from build123d import *
from build123d.topology import SkipClean

# Parameters (mm, degrees)
SKETCH_1_W                 = 85
SKETCH_1_H                 = 5
EXTRUDE_1_DEPTH            = 8
EXTRUDE_1_2_DEPTH          = 8
SKETCH_1_3_W               = 85
SKETCH_1_3_H               = 20
EXTRUDE_2_DEPTH            = 11
EXTRUDE_3_DEPTH            = 21
SKETCH_6_R                 = 6.5
SKETCH_6_R_2               = 4
CUT_EXTRUDE_1_DEPTH        = 3
SKETCH_6_2_R               = 4
CUT_EXTRUDE_2_DEPTH        = 21
EXTRUDE_6_DEPTH            = 20
EXTRUDE_7_DEPTH            = 15
SKETCH_10_4_W              = 15
SKETCH_10_4_H              = 4
CUT_EXTRUDE_4_DEPTH        = 15
CUT_EXTRUDE_2_2_DEPTH      = 66.048059256
CUT_EXTRUDE_2_2_DEPTH_BACK = 1
CUT_EXTRUDE_2_2_START      = 25
SKETCH_12_W                = 2
SKETCH_12_H                = 40
CUT_EXTRUDE_5_REACH        = 59.985
SKETCH_6_4_R               = 4
CUT_EXTRUDE_6_DEPTH        = 81.357015954


with BuildPart() as part:
    # Sketch 1 → Extrude 1 (new body)
    with BuildSketch(Plane(origin=(0, 0, 0), x_dir=(1, 0, 0), z_dir=(0, 1, 0))):
        with Locations((0, 12.5)):
            Rectangle(SKETCH_1_W, SKETCH_1_H)
    extrude(amount=EXTRUDE_1_DEPTH)



with BuildPart() as body_2:
    # Sketch 1 → Extrude 1 2 (new body)
    with BuildSketch(Plane(origin=(0, 0, 0), x_dir=(1, 0, 0), z_dir=(0, 1, 0))):
        with Locations((0, -12.5)):
            Rectangle(SKETCH_1_W, SKETCH_1_H)
    extrude(amount=EXTRUDE_1_2_DEPTH)


with BuildPart() as part_1:
    add(part.part)

    add(body_2.part)  # Extrude 2 merges body 2
    # Sketch 1_3 → Extrude 2 (add)
    with BuildSketch(Plane(origin=(0, 0, 0), x_dir=(1, 0, 0), z_dir=(0, 1, 0))):
        Rectangle(SKETCH_1_3_W, SKETCH_1_3_H)
    extrude(amount=EXTRUDE_2_DEPTH)

    # Sketch 3 → Extrude 3 (add, symmetric)
    with BuildSketch(Plane(origin=(0, 0, 0), x_dir=(0, 0, -1), z_dir=(1, 0, 0))):
        with BuildLine():
            Line((-10, 35), (-10, 11))
            Line((-10, 11), (10, 11))
            Line((10, 11), (10, 35))
            ThreePointArc((10, 35), (0, 45), (-10, 35))
        make_face()
    extrude(amount=EXTRUDE_3_DEPTH, both=True)

    # Sketch 6 → Cut-Extrude 1 (cut)
    with BuildSketch(Plane.ZY.offset(21)):
        with Locations((0, 35)):
            Circle(SKETCH_6_R)
        with Locations((0, 35)):
            Circle(SKETCH_6_R_2, mode=Mode.SUBTRACT)
    cut_extrude_1 = extrude(amount=-CUT_EXTRUDE_1_DEPTH, mode=Mode.SUBTRACT)

    # Sketch 6_2 → Cut-Extrude 2 (cut)
    with BuildSketch(Plane.ZY.offset(21)):
        with Locations((0, 35)):
            Circle(SKETCH_6_2_R)
    cut_extrude_2 = extrude(amount=-CUT_EXTRUDE_2_DEPTH, mode=Mode.SUBTRACT)

    # Mirror 1: Cut-Extrude 1, Cut-Extrude 2 across plane
    add(cut_extrude_1.mirror(Plane(origin=(0, 0, 0), x_dir=(0, 0, 1), z_dir=(1, 0, 0))), mode=Mode.SUBTRACT)
    add(cut_extrude_2.mirror(Plane(origin=(0, 0, 0), x_dir=(0, 0, 1), z_dir=(1, 0, 0))), mode=Mode.SUBTRACT)

    # Sketch 10 → Extrude 6 (add, symmetric)
    with SkipClean():  # the faces are left unmerged after this step: merging them gives an invalid solid
        with BuildSketch(Plane.XY):
            with BuildLine():
                ThreePointArc((15, 25), (10.606601718, 35.606601718), (0, 40))
                Line((0, 40), (0, 33))
                ThreePointArc((0, 33), (5.656854249, 30.656854249), (8, 25))
                ThreePointArc((8, 25), (5.656854249, 19.343145751), (0, 17))
                Line((0, 17), (0, 10))
                ThreePointArc((0, 10), (10.606601718, 14.393398282), (15, 25))
            make_face()
            with BuildLine():
                Line((0, 33), (0, 40))
                ThreePointArc((0, 40), (-10.606601718, 35.606601718), (-15, 25))
                ThreePointArc((-15, 25), (-10.606601718, 14.393398282), (0, 10))
                Line((0, 10), (0, 17))
                ThreePointArc((0, 17), (-8, 25), (0, 33))
            make_face()
        extrude(amount=EXTRUDE_6_DEPTH, both=True)
    add(part_1.part.scale(1), mode=Mode.REPLACE)  # the faces are merged on a copy

    # Sketch 10_3 → Extrude 7 (add, symmetric)
    with BuildSketch(Plane.XY):
        with BuildLine():
            Line((15, 8), (15, 25))
            ThreePointArc((15, 25), (10.606601718, 14.393398282), (0, 10))
            Line((0, 10), (0, 8))
            Line((0, 8), (15, 8))
        make_face()
        with BuildLine():
            ThreePointArc((0, 10), (-10.606601718, 14.393398282), (-15, 25))
            Line((-15, 25), (-15, 8))
            Line((-15, 8), (0, 8))
            Line((0, 8), (0, 10))
        make_face()
    extrude(amount=EXTRUDE_7_DEPTH, both=True)

    # Sketch 10_4 → Cut-Extrude 4 (cut, symmetric)
    with BuildSketch(Plane.XY):
        with BuildLine():
            ThreePointArc((8, 25), (5.656854249, 30.656854249), (0, 33))
            Line((0, 33), (0, 17))
            ThreePointArc((0, 17), (5.656854249, 19.343145751), (8, 25))
        make_face()
        with BuildLine():
            Line((0, 17), (0, 33))
            ThreePointArc((0, 33), (-8, 25), (0, 17))
        make_face()
        with Locations((-7.5, 2)):
            Rectangle(SKETCH_10_4_W, SKETCH_10_4_H)
        with Locations((7.5, 2)):
            Rectangle(SKETCH_10_4_W, SKETCH_10_4_H)
    extrude(amount=CUT_EXTRUDE_4_DEPTH, both=True, mode=Mode.SUBTRACT)

    # Sketch 12 → Cut-Extrude 2 2 (cut, two sides: drawn at the far end of the back side and taken through both)
    with BuildSketch(Plane(origin=(0, 0, 0), x_dir=(1, 0, 0), z_dir=(0, 1, 0)).offset(CUT_EXTRUDE_2_2_START - CUT_EXTRUDE_2_2_DEPTH_BACK)):
        Rectangle(SKETCH_12_W, SKETCH_12_H)
    extrude(amount=CUT_EXTRUDE_2_2_DEPTH + CUT_EXTRUDE_2_2_DEPTH_BACK, mode=Mode.SUBTRACT)

    # Sketch 14 → Cut-Extrude 5 (cut, up to next)
    with BuildSketch(Plane(origin=(0, 11, 0), x_dir=(1, 0, 0), z_dir=(0, 1, 0)), mode=Mode.PRIVATE) as cut_extrude_5_sk1:
        with BuildLine():
            Line((-35, 4), (-30, 4))
            ThreePointArc((-30, 4), (-26, 0), (-30, -4))
            Line((-30, -4), (-35, -4))
            ThreePointArc((-35, -4), (-39, 0), (-35, 4))
        make_face()
    cut_extrude_5_tool1 = extrude(cut_extrude_5_sk1.sketch, amount=-CUT_EXTRUDE_5_REACH, mode=Mode.PRIVATE) & part_1.part
    # Sketch 14 → Cut-Extrude 5 (cut, up to next)
    with BuildSketch(Plane(origin=(0, 11, 0), x_dir=(1, 0, 0), z_dir=(0, 1, 0)), mode=Mode.PRIVATE) as cut_extrude_5_sk2:
        with BuildLine():
            Line((35, 4), (30, 4))
            ThreePointArc((30, 4), (26, 0), (30, -4))
            Line((30, -4), (35, -4))
            ThreePointArc((35, -4), (39, 0), (35, 4))
        make_face()
    cut_extrude_5_tool2 = extrude(cut_extrude_5_sk2.sketch, amount=-CUT_EXTRUDE_5_REACH, mode=Mode.PRIVATE) & part_1.part
    add(cut_extrude_5_tool1.solids().sort_by_distance((-32.5, 11, 0))[0], mode=Mode.SUBTRACT)
    add(cut_extrude_5_tool2.solids().sort_by_distance((32.5, 11, 0))[0], mode=Mode.SUBTRACT)

    # Sketch 6_4 → Cut-Extrude 6 (cut, through all)
    with BuildSketch(Plane.ZY.offset(21)):
        with Locations(Location((0, 35, 0), (0, 0, 328.956646236))):
            Circle(SKETCH_6_4_R)
    extrude(amount=-CUT_EXTRUDE_6_DEPTH, mode=Mode.SUBTRACT)


solid = part_1.part
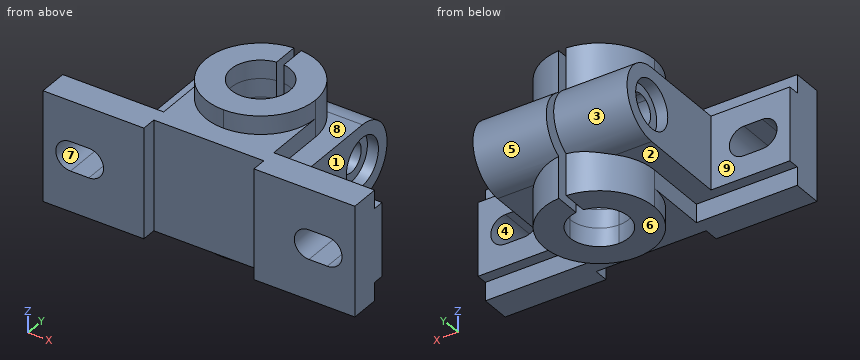
The listing builds one solid part. Answer for the finished solid, in the listing's coordinates (mm). Face numbers are marked on the shaded views. A direction names the side the tool comes from. Round coordinates to 2 decimals unless told otherwise and drop trailing zeros. Order: outer loops, then holes, each group sorted by start corner. A loop starts at its lowest first (then second) coordinate and runs counter-clockwise, first axis right, second up. Notation, with made-up numbers: (1, -29.5) -> (25, -29.5) arc R18 ccw to (25, -2.5) -> close; hole circle Ø6 at (10.25, 89). An arc over 180 degrees is marked (long way). Write each question's results on one line, items separated by ' | '. Start each with the question number.
Q1. Straight lines are drawn through the part: probe 1 along X at (y, z) = (36, -7.5); probe 2 along X at (y, z) = (35, 4.5); probe 3 along Y at (x, z) = (-9, 0). For each, find the intervals that lie inside material, in ascending order. Write a range as from..to.
Q2. Find section A-A (y = 3). Determine the outline of the cut face in (x, z).
Q3. Find section D-D (y = 38). Give the number of separate pieces and of enclosed holes in the cut face, then the cut area to 3 significant figures.
Q4. The mould has two halves that part along Z. Classify the marked faces 6, 7, 8 and 9: pulls with the +Z half, pulls with the -Z half, needs draft (parallel to the pull), parting line crosses it, or undercut.
Q5. Find section B-B (x = 16). Determine the outline of the cut face in (y, z), then the cut area to 3 significant figures.
Q6. Each of these flat-tipped pins is pushed along its axis until it touches: pin 1 (1 mm diameter, centred on y = 33, z = 14.5, fed in from -X); pin 2 (4 mm diameter, centred on x = 22, y = 11, fed in from +Z); pin 3 (10 mm diameter, centred on y = 21.5, z = 6.5, fed in from -X). Where does it stop, or does it pass through?
Q7. Which of the six approach directions +Z, -Z, +X, -X, +Y, -Y give full straight-line access (tool end or side, diameter ignored) to the marked faces 1, 2, 3, 4 and 5?
Worked answers:
1) probe 1: x = -21..-1, 1..21 | probe 2: x = -18..-1, 1..18 | probe 3: y = 4..31, 39..45
2) outline: (-42.5, -15) -> (-15, -15) -> (-15, 15) -> (-42.5, 15) -> close; (15, -15) -> (42.5, -15) -> (42.5, 15) -> (15, 15) -> close; hole (-35, -4) -> (-30, -4) arc R4 ccw to (-30, 4) -> (-35, 4) arc R4 ccw to start; hole (30, -4) -> (35, -4) arc R4 ccw to (35, 4) -> (30, 4) arc R4 ccw to start
3) separate pieces: 4 | enclosed holes: 0 | area: 785 mm2
4) face 6: pulls with the -Z half | face 7: undercut | face 8: pulls with the +Z half | face 9: needs draft
5) outline: (0, -15) -> (8, -15) -> (8, -10) -> (35, -10) arc R10 ccw to (35, 10) -> (8, 10) -> (8, 15) -> (0, 15) -> close; hole circle Ø8 at (35, 0) | area: 887 mm2
6) pin 1: stops at x = -12.99 | pin 2: stops at z = 10 | pin 3: stops at x = -21
7) face 1: +Z, -Z, +X, +Y | face 2: -Z, -X, +Y | face 3: -X, +Y | face 4: +Y, -Y | face 5: +X, +Y
